Build history of the part. All positions in model axes, mm. Give positions to 0.01 mm unless a question says otherwise; leave off trailing zeros. Order: outer loops, then holes, each group sorted by start corner. A loop starts at its lowest first (then second) coordinate and runs counter-clockwise, first axis right, second up. Notation, with made-up numbers: M -8,-14.75 L 19,-14.75 A7 cw 19,-4.75 Z; hole C 35,49 d9. An arc over 180 degrees is marked long. Use CSV: the item, a comma, the result in double quotes. Start each with the question number.
Item 1: Band-saw the part on C-C on y = 105. Write the cut outline in (x, z) (3 decimals).
Item 2: Pin check, flat tip, straight feed: P1, Ø0.5, axis at x = 203.5, z = 0.5, coming from the -Y side. Stop position of the tip, or through.
Item 3: Wall check: line 1 along X through (y, z) = (136, 0.75); line 2 along Y through (x, z) = (175, 0.85) (3 decimals). Give the ranges that are in metal, low to high.
Item 4: Band-saw the part on A-A on x = 235. Write the cut outline in (y, z), plus the area to 3 significant figures.
Item 5: Band-saw the part on D-D on z = 0.2. Give the number of separate pieces and of enclosed holes in the cut face, plus the area to 3 significant figures.
from build123d import *

# Parameters (mm, degrees)
ESQUISSE1_R        = 3.175
ESQUISSE1_W        = 60
ESQUISSE1_H        = 60
BOSS_EXTRU_1_DEPTH = 1


with BuildPart() as part:
    # Esquisse1 → Boss.-Extru.1 (new body)
    with BuildSketch(Plane.XY):
        Polygon((110, 310), (100, 310), (100, 250), (40, 250), (40, 240), (100, 240), (100, 180), (40, 180), (40, 170), (100, 170), (100, 110), (40, 110), (40, 100), (100, 100), (100, 40), (110, 40), (110, 100), (170, 100), (170, 40), (180, 40), (180, 100), (240, 100), (240, 40), (250, 40), (250, 100), (310, 100), (310, 110), (250, 110), (250, 170), (310, 170), (310, 180), (250, 180), (250, 240), (310, 240), (310, 250), (250, 250), (250, 310), (240, 310), (240, 250), (180, 250), (180, 310), (170, 310), (170, 250), (110, 250), align=None)
        with Locations((105, 105)):
            Circle(ESQUISSE1_R, mode=Mode.SUBTRACT)
        with Locations((140, 140)):
            Rectangle(ESQUISSE1_W, ESQUISSE1_H, mode=Mode.SUBTRACT)
        with Locations((105, 175)):
            Circle(ESQUISSE1_R, mode=Mode.SUBTRACT)
        with Locations((140, 210)):
            Rectangle(ESQUISSE1_W, ESQUISSE1_H, mode=Mode.SUBTRACT)
        with Locations((105, 245)):
            Circle(ESQUISSE1_R, mode=Mode.SUBTRACT)
        with Locations((175, 245)):
            Circle(ESQUISSE1_R, mode=Mode.SUBTRACT)
        with Locations((175, 105)):
            Circle(ESQUISSE1_R, mode=Mode.SUBTRACT)
        with Locations((210, 140)):
            Rectangle(ESQUISSE1_W, ESQUISSE1_H, mode=Mode.SUBTRACT)
        with Locations((245, 105)):
            Circle(ESQUISSE1_R, mode=Mode.SUBTRACT)
        with Locations((175, 175)):
            Circle(ESQUISSE1_R, mode=Mode.SUBTRACT)
        with Locations((210, 210)):
            Rectangle(ESQUISSE1_W, ESQUISSE1_H, mode=Mode.SUBTRACT)
        with Locations((245, 175)):
            Circle(ESQUISSE1_R, mode=Mode.SUBTRACT)
        with Locations((245, 245)):
            Circle(ESQUISSE1_R, mode=Mode.SUBTRACT)
    extrude(amount=BOSS_EXTRU_1_DEPTH)


solid = part.part
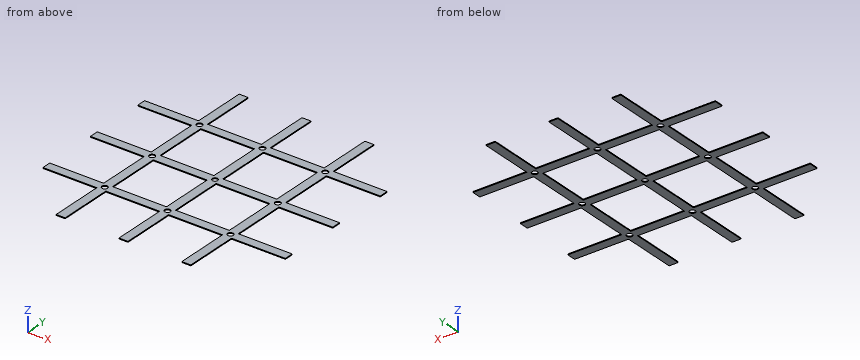
Model answer:
1,outline,"M 40,0 L 101.825,0 L 101.825,1 L 40,1 Z; M 108.175,0 L 171.825,0 L 171.825,1 L 108.175,1 Z; M 178.175,0 L 241.825,0 L 241.825,1 L 178.175,1 Z; M 248.175,0 L 310,0 L 310,1 L 248.175,1 Z"
2,P1,"stops at y = 100"
3,line 1,"x = 100 to 110, 170 to 180, 240 to 250"
3,line 2,"y = 40 to 101.825, 108.175 to 171.825, 178.175 to 241.825, 248.175 to 310"
4,outline,"M 100,0 L 110,0 L 110,1 L 100,1 Z; M 170,0 L 180,0 L 180,1 L 170,1 Z; M 240,0 L 250,0 L 250,1 L 240,1 Z"
4,area,"30.0 mm^2"
5,separate pieces,"1"
5,enclosed holes,"13"
5,area,"15,000 mm^2"
